The figure shows three views and two pictorial views of one solid part (mm, origin at its lowest corner). Answer the questions. Coordinates: 2 decimals unless noted, no trailing zeros. Write each loop counter-clockwise with the first axis right and the second up, starting at its lowest first coordinate (ties: lowest second). Pieces come first, ordered by that corner, then holes.
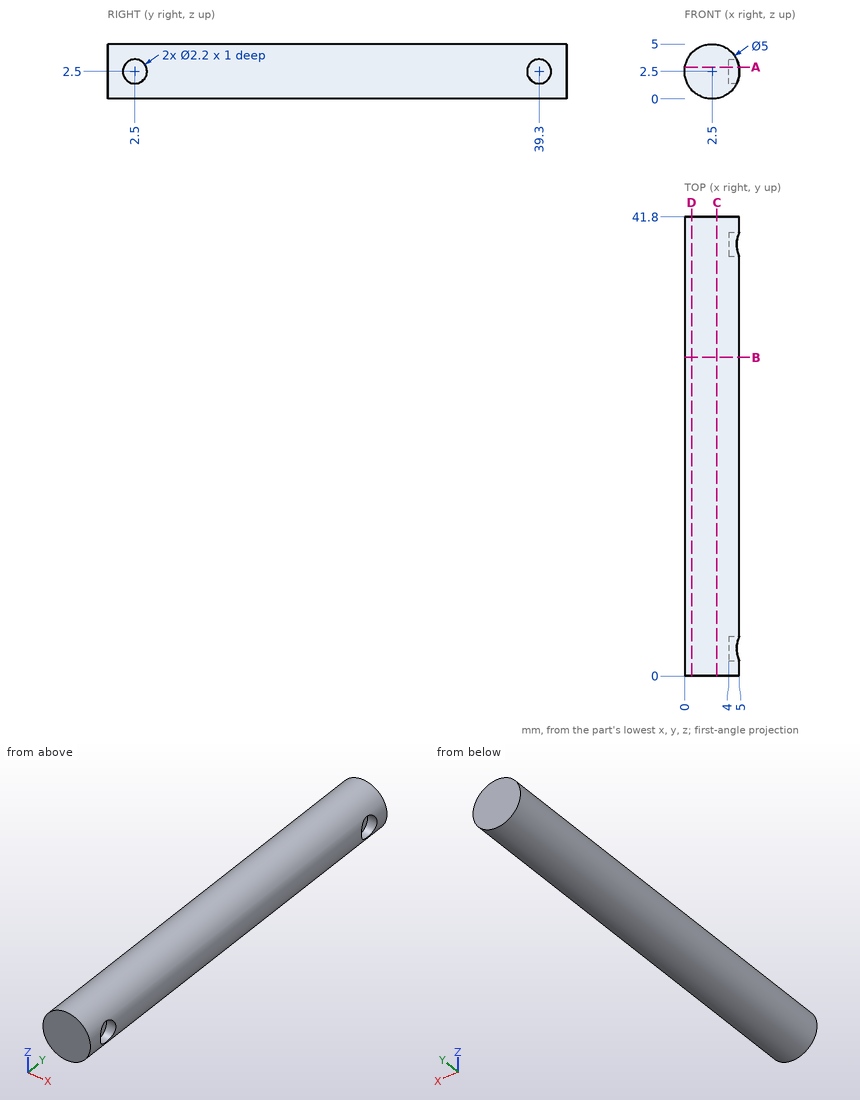
1. Section B-B on y = 29 is taken. Give the vertices of the cut face in (x, z), then the cut area to 3 significant figures.
Results found:
outline: circle Ø5 at (2.5, 2.5)
area: 19.6 mm2
2. Section D-D on x = 0.65 is taken. Give the vertices of the cut face in (y, z), then the cut area to 3 significant figures.
Results found:
outline: (0, 0.82) - (41.8, 0.82) - (41.8, 4.18) - (0, 4.18) - close
area: 141 mm2
3. Section C-C on x = 2.95 is taken. Give the vertices of the cut face in (y, z).
Results found:
outline: (0, 0.04) - (41.8, 0.04) - (41.8, 4.96) - (0, 4.96) - close
4. Flat-ended cylindrical pins translate along their axes: P1, Ø2, axis at x = 0.5, y = 28.5, coming from the -Z side; P2, Ø0.7, axis at y = 39, z = 2, coming from the +X side; P3, Ø1.5, axis at y = 35, z = 1, coming from the -X side. Find the tip coordinate at first contact, or state that the pin passes through.
Results found:
P1: stops at z = 0.21
P2: stops at x = 4
P3: stops at x = 0.12
5. Find the intervals of material crossed by L1, parallel to Y at x = 4.3, z = 2.5; L2, parallel to Z at x = 2.65, y = 30; L3, parallel to Z at x = 3.45, y = 37, in increasing order.
Results found:
L1: y = 0 to 1.4, 3.6 to 38.2, 40.4 to 41.8
L2: z = 0 to 5
L3: z = 0.19 to 4.81
6. Section A-A on z = 2.9 is taken. Give the vertices of the cut face in (x, y), then the cut area to 3 significant figures.
Results found:
outline: (0.03, 0) - (4.97, 0) - (4.97, 1.48) - (4, 1.48) - (4, 3.52) - (4.97, 3.52) - (4.97, 38.28) - (4, 38.28) - (4, 40.32) - (4.97, 40.32) - (4.97, 41.8) - (0.03, 41.8) - close
area: 202 mm2
